```python
from build123d import *

# Parameters (mm, degrees)
SALIENTE_EXTRUIR1_START     = -14.8
SALIENTE_EXTRUIR1_OUTLINE_W = 17.2
SALIENTE_EXTRUIR1_OUTLINE_H = 14
SALIENTE_EXTRUIR1_DEPTH     = 15.6
CROQUIS2_W                  = 14
CROQUIS2_H                  = 14.8
SALIENTE_EXTRUIR2_DEPTH     = 0.8
CROQUIS3_W                  = 18
CROQUIS3_H                  = 7
SALIENTE_EXTRUIR3_DEPTH     = 3.2
CROQUIS4_W                  = 8
CROQUIS4_H                  = 3
CORTAR_EXTRUIR1_DEPTH       = 25.515301344
TALADRO1_D                  = 10
CHAFL_N1_SIZE               = 0.7
CROQUIS7_W                  = 7
CROQUIS7_H                  = 3.2
CORTAR_EXTRUIR2_DEPTH       = 23.6
CROQUIS8_W                  = 8
CROQUIS8_H                  = 0.599553283
SALIENTE_EXTRUIR4_DEPTH     = 18
CROQUIS9_W                  = 8
CROQUIS9_H                  = 3
CORTAR_EXTRUIR3_DEPTH       = 23.3
CROQUIS10_W                 = 8
CROQUIS10_H                 = 18
SALIENTE_EXTRUIR5_DEPTH     = 18
CROQUIS11_OUTSIDE_W         = 26.014
CROQUIS11_OUTSIDE_H         = 26.014
CROQUIS11_OUTSIDE_W_2       = 15
CROQUIS11_OUTSIDE_H_2       = 18
CORTAR_EXTRUIR4_DEPTH       = 30.1
CHAFL_N3_SIZE               = 0.8
CROQUIS12_R                 = 5
CORTAR_EXTRUIR5_DEPTH       = 30.1


with BuildPart() as part:
    # Saliente-Extruir1: read off the stored shape, not the designer's step
    # Saliente-Extruir1 outline → Saliente-Extruir1 (new body)
    with BuildSketch(Plane.XZ.offset(5.8).offset(SALIENTE_EXTRUIR1_START)):
        with Locations((0.4, -7)):
            Rectangle(SALIENTE_EXTRUIR1_OUTLINE_W, SALIENTE_EXTRUIR1_OUTLINE_H)
    extrude(amount=SALIENTE_EXTRUIR1_DEPTH)

    # Saliente-Extruir1 2 outline → Saliente-Extruir1 2 (revolve, cut)
    with BuildSketch(Plane(origin=(-7.4, 0, -3.5), x_dir=(1, 0, 0), z_dir=(0, 0, 1))):
        with BuildLine():
            Line((19.473315075, -5.8), (0.8, -5.799999999))
            ThreePointArc((0.8, -5.799999999), (0.565685425, -6.365685425), (0, -6.6))
            Line((0, -6.6), (19.473315075, -6.6))
            Line((19.473315075, -6.6), (19.473315075, -5.8))
        make_face()
    revolve(axis=Axis((-7.4, 0, -3.5), (0, 1, 0)), mode=Mode.SUBTRACT)

    # Croquis2 → Saliente-Extruir2 (add)
    with BuildSketch(Plane.ZY.offset(8.2)):
        with Locations((-7, 1.6)):
            Rectangle(CROQUIS2_W, CROQUIS2_H)
    extrude(amount=SALIENTE_EXTRUIR2_DEPTH)

    # Croquis3 → Saliente-Extruir3 (add)
    with BuildSketch(Plane.XZ.offset(5.8)):
        with Locations((0, -10.5)):
            Rectangle(CROQUIS3_W, CROQUIS3_H)
    extrude(amount=SALIENTE_EXTRUIR3_DEPTH)

    # Croquis4 → Cortar-Extruir1 (cut, through all)
    with BuildSketch(Plane.ZY.offset(9)):
        with Locations((-4, 7.5)):
            Rectangle(CROQUIS4_W, CROQUIS4_H)
    extrude(amount=-CORTAR_EXTRUIR1_DEPTH, mode=Mode.SUBTRACT)

    # Taladro1 (through all)
    with Locations(Plane(origin=(0, 0, -14), x_dir=(-1, 0, 0), z_dir=(0, 0, -1))):
        with Locations((0, 0)):
            Hole(TALADRO1_D / 2)

    # Chaflán1
    chafl_n1_edges = [part.edges().sort_by_distance(p)[0] for p in [
        (0, 9, -14),
        (0, -9, -14),
    ]]
    chamfer(chafl_n1_edges, length=CHAFL_N1_SIZE)

    # Croquis7 → Cortar-Extruir2 (cut)
    with BuildSketch(Plane(origin=(9, 0, 0), x_dir=(0, 0, -1), z_dir=(1, 0, 0))):
        with Locations((3.5, -7.4)):
            Rectangle(CROQUIS7_W, CROQUIS7_H)
    extrude(amount=-CORTAR_EXTRUIR2_DEPTH, mode=Mode.SUBTRACT)

    # Croquis8 → Saliente-Extruir4 (add)
    with BuildSketch(Plane.ZY.offset(9)):
        with Locations((-4, -5.700223359)):
            Rectangle(CROQUIS8_W, CROQUIS8_H)
    extrude(amount=-SALIENTE_EXTRUIR4_DEPTH)

    # Croquis9 → Cortar-Extruir3 (cut)
    with BuildSketch(Plane.ZY.offset(9)):
        with Locations((-4, -7.5)):
            Rectangle(CROQUIS9_W, CROQUIS9_H)
    extrude(amount=-CORTAR_EXTRUIR3_DEPTH, mode=Mode.SUBTRACT)

    # Croquis10 → Saliente-Extruir5 (add)
    with BuildSketch(Plane.ZY.offset(9)):
        with Locations((-12, 0)):
            Rectangle(CROQUIS10_W, CROQUIS10_H)
    extrude(amount=-SALIENTE_EXTRUIR5_DEPTH)

    # Croquis11 outside → Cortar-Extruir4 (cut)
    with BuildSketch(Plane.XY):
        Rectangle(CROQUIS11_OUTSIDE_W, CROQUIS11_OUTSIDE_H)
        Rectangle(CROQUIS11_OUTSIDE_W_2, CROQUIS11_OUTSIDE_H_2, mode=Mode.SUBTRACT)
    extrude(amount=-CORTAR_EXTRUIR4_DEPTH, mode=Mode.SUBTRACT)

    # Chaflán3
    chafl_n3_edges = [part.edges().sort_by_distance(p)[0] for p in [
        (0, 9, -16),
        (0, -9, -16),
        (0, -9, -8),
        (0, -6, 0),
        (0, 9, -8),
        (0, 6, 0),
        (-7.5, 0, 0),
        (7.5, 0, 0),
    ]]
    chamfer(chafl_n3_edges, length=CHAFL_N3_SIZE)

    # Croquis12 → Cortar-Extruir5 (cut)
    with BuildSketch(Plane.XY.offset(-8)):
        with Locations(Location((0, 0, 0), (0, 0, 90))):
            Circle(CROQUIS12_R)
    extrude(amount=-CORTAR_EXTRUIR5_DEPTH, mode=Mode.SUBTRACT)


solid = part.part
```
Geometry: final body of the model. Coordinates: model frame, mm. A direction names the side the tool comes from. Round coordinates to 2 decimals unless told otherwise and drop trailing zeros. Write each loop counter-clockwise with the first axis right and the second up, starting at its lowest first coordinate (ties: lowest second). Pieces come first, ordered by that corner, then holes. Notation, with made-up numbers: (20.5, 63) -> (62.5, 63) arc R22 cw to (62.5, 93) -> close; hole circle Ø2 at (28.5, 37.25). An arc over 180 degrees is marked (long way). Return JSON: item names as keys, results as strings.
Q1. Section B-B on y = -3. Return the cut outline in (x, z), and give its area (3 significant figures).
From the geometry:
{"outline": "(-7.5, -16) -> (-4, -16) -> (-4, 0) -> (-6.7, 0) -> (-7.5, -0.8) -> close; (4, -16) -> (7.5, -16) -> (7.5, -0.8) -> (6.7, 0) -> (4, 0) -> close", "area": "111 mm2"}
Q2. First-contact query: pin 1 Ø1.8 at (x, y) = (-3, 6.5) entering from +Z; pin 2 Ø2 at (x, z) = (-1.5, -6) entering from -Y; pin 3 Ø8 at (x, y) = (0, 0) entering from -Z; pin 4 Ø2 at (x, z) = (2.5, -3.5) entering from +Y. Flat tips, straight axial feed; report the tip coordinate or a pass-through.
From the geometry:
{"pin 1": "z = -0.4", "pin 2": "y = -6", "pin 3": "through", "pin 4": "y = 6"}
Q3. Section A-A on x = -4. Return the cut outline in (y, z), and give its area (3 significant figures).
From the geometry:
{"outline": "(-9, -15.2) -> (-8.2, -16) -> (-3, -16) -> (-3, 0) -> (-5.2, 0) -> (-6, -0.8) -> (-6, -8) -> (-8.2, -8) -> (-9, -8.8) -> close; (3, -16) -> (8.2, -16) -> (9, -15.2) -> (9, -8.8) -> (8.2, -8) -> (6, -8) -> (6, -0.8) -> (5.2, 0) -> (3, 0) -> close", "area": "142 mm2"}
Q4. Mould query, pull axis X, two halves, no side actions, for faces 1 (the flat face through (-7.5, 0, -8)), 2 (the flat face through (-0.1, 8.6, -15.6)), 3 (the cylindrical face through (4.64, 1.86, -7.89)). Classes: +X half, -X half, draft (parallel to the pull), parting line (faces both ways), or undercut.
From the geometry:
{"face 1": "-X half", "face 2": "draft", "face 3": "undercut"}
Q5. Section C-C on x = 5.5. Return the cut outline in (y, z).
From the geometry:
{"outline": "(-9, -15.2) -> (-8.2, -16) -> (8.2, -16) -> (9, -15.2) -> (9, -8.8) -> (8.2, -8) -> (6, -8) -> (6, -0.8) -> (5.2, 0) -> (-5.2, 0) -> (-6, -0.8) -> (-6, -8) -> (-8.2, -8) -> (-9, -8.8) -> close"}
Q6. Ray query, line 1 (Y direction, x = 0, z = -7); line 2 (X direction, y = 0, z = -9); line 3 (Z direction, x = -4.25, y = 7.75). Return the intervals inside material, ascending.
From the geometry:
{"line 1": "-6 to -5, 5 to 6", "line 2": "-7.5 to -5, 5 to 7.5", "line 3": "-16 to -8"}
Q7. Section D-D on z = -1.75. Return the cut outline in (x, y).
From the geometry:
{"outline": "(-7.5, -6) -> (7.5, -6) -> (7.5, 6) -> (-7.5, 6) -> close; hole circle Ø10 at (0, 0)"}
Q8. Set-up query: faces 4 (the flat face through (0, -6, -4)), 5 (the flat face through (0, 7, -8)), 6 (the flat face through (0, 9, -12)). Return all of +Z, -Z, +X, -X, +Y, -Y with unobstructed straight access to the full face (end or side cutting, diameter ignored); none if empty.
From the geometry:
{"face 4": "+Z, +X, -X, -Y", "face 5": "+Z, +X, -X, +Y", "face 6": "+Z, -Z, +X, -X, +Y"}
